Verification items for this drawing (mm, ordinates from the low corner). Coordinates: 2 decimals unless noted, no trailing zeros. Write each loop counter-clockwise with the first axis right and the second up, starting at its lowest first coordinate (ties: lowest second). Pieces come first, ordered by that corner, then holes. Notation, with made-up numbers: M -16,75.5 L 4,75.5 A4 cw 4,80.5 Z; hole C 57,42 d8. An arc over 180 degrees is marked long. Answer as CSV lines item,"result". Start each with the question number.
1) Section check D-D (x = 106). Record the cut outline in (y, z).
2) Material ranges on L1, parallel to Y at x = 56.6, z = 2.7; L2, parallel to Y at x = 68.4, z = 1.25; L3, parallel to X at y = 112, z = 1.7, recorded low to high. Write a range as [from, to].
3) Go/stop test with flat-tipped pins: pin 1 Ø1 at (y, z) = (98.5, 1) entering from +X; pin 2 Ø1 at (y, z) = (35, 0.5) entering from -X; pin 3 Ø1.5 at (y, z) = (44, 0.5) entering from +X. Record where each tip stops, or that it passes through.
4) Section check A-A (x = 56.6). Record the cut outline in (y, z), and give its area (3 significant figures).
5) Section check B-B (z = 0.8). Record the cut outline in (x, y).
6) Section check C-C (y = 93). Record the cut outline in (x, z).
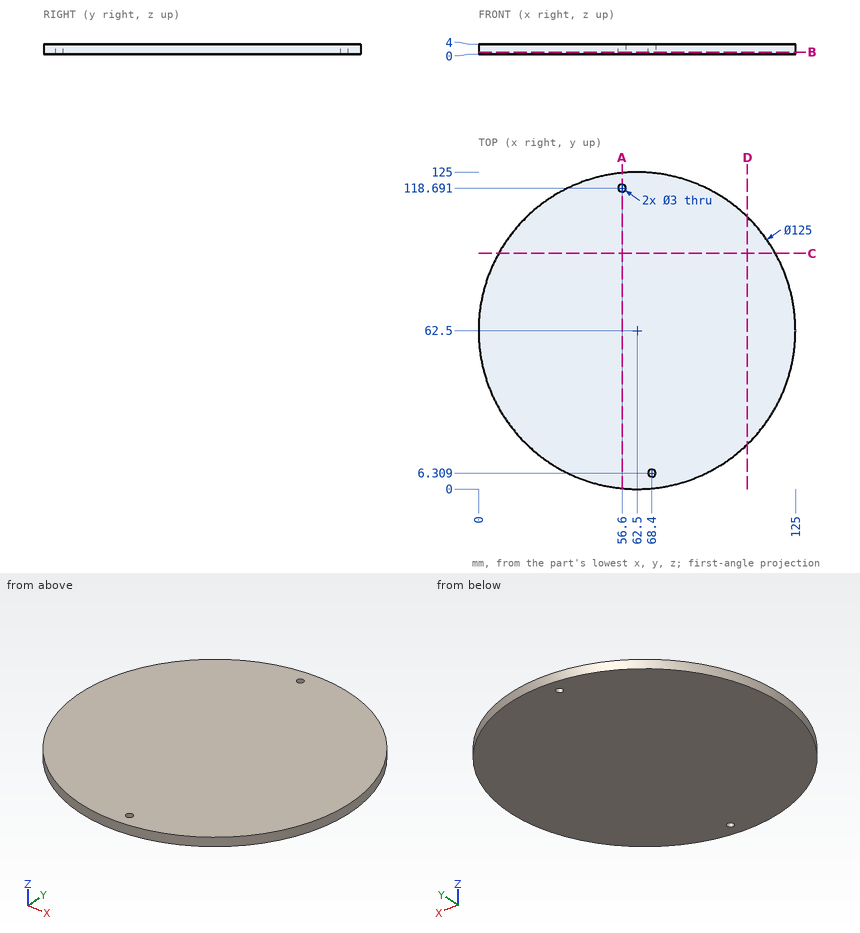
Results found:
1,outline,"M 17.62,0 L 107.38,0 L 107.38,4 L 17.62,4 Z"
2,L1,"y = [0.28, 117.19], [120.19, 124.72]"
2,L2,"y = [0.28, 4.81], [7.81, 124.72]"
2,L3,"x = [24.34, 100.66]"
3,pin 1,"stops at x = 113.94"
3,pin 2,"stops at x = 6.13"
3,pin 3,"stops at x = 122.43"
4,outline,"M 0.28,0 L 117.19,0 L 117.19,4 L 0.28,4 Z; M 120.19,0 L 124.72,0 L 124.72,4 L 120.19,4 Z"
4,area,"486 mm2"
5,outline,"C 62.5,62.5 d125; hole C 56.6,118.69 d3; hole C 68.4,6.31 d3"
6,outline,"M 7.95,0 L 117.05,0 L 117.05,4 L 7.95,4 Z"
